from build123d import *

# Parameters (mm, degrees)
BOSS_EXTRUDE1_DEPTH            = 40.64
F_31_0_12_DIAMETER_HOLE2_D     = 3.048
F_31_0_12_DIAMETER_HOLE2_DEPTH = 12.7
F_31_0_12_DIAMETER_HOLE2_TIP   = 0.915711583
F_31_0_12_DIAMETER_HOLE1_D     = 3.048
F_31_0_12_DIAMETER_HOLE1_DEPTH = 12.7
F_31_0_12_DIAMETER_HOLE1_TIP   = 0.915711583
CHAMFER1_SIZE                  = 31.75


with BuildPart() as part:
    # Sketch1 → Boss-Extrude1 (new, symmetric)
    with BuildSketch(Plane.XY):
        Polygon((48.0568, 17.74825), (-48.0568, 17.74825), (-48.0568, -17.74825), (-40.132, -17.74825), (-40.132, 12.98575), (40.132, 12.98575), (40.132, -17.74825), (48.0568, -17.74825), align=None)
    extrude(amount=BOSS_EXTRUDE1_DEPTH, both=True)

    # #31 (0.12) Diameter Hole2
    with Locations(Plane(origin=(0, -17.74825, 0), x_dir=(-1, 0, 0), z_dir=(0, -1, 0))):
        with Locations((-44.0944, 0), (44.0944, 0)):
            Hole(F_31_0_12_DIAMETER_HOLE2_D / 2, depth=F_31_0_12_DIAMETER_HOLE2_DEPTH)
            with Locations((0, 0, -(F_31_0_12_DIAMETER_HOLE2_DEPTH + F_31_0_12_DIAMETER_HOLE2_TIP / 2))):  # 118° drill point
                Cone(0, F_31_0_12_DIAMETER_HOLE2_D / 2, F_31_0_12_DIAMETER_HOLE2_TIP, mode=Mode.SUBTRACT)

    # #31 (0.12) Diameter Hole1
    with Locations(Plane(origin=(0, 17.74825, 0), x_dir=(1, 0, 0), z_dir=(0, 1, 0))):
        with Locations((0, -36.83), (0, 36.83)):
            Hole(F_31_0_12_DIAMETER_HOLE1_D / 2, depth=F_31_0_12_DIAMETER_HOLE1_DEPTH)
            with Locations((0, 0, -(F_31_0_12_DIAMETER_HOLE1_DEPTH + F_31_0_12_DIAMETER_HOLE1_TIP / 2))):  # 118° drill point
                Cone(0, F_31_0_12_DIAMETER_HOLE1_D / 2, F_31_0_12_DIAMETER_HOLE1_TIP, mode=Mode.SUBTRACT)

    # Chamfer1
    chamfer1_edges = [part.edges().sort_by_distance(p)[0] for p in [
        (-48.0568, 0, 40.64),
        (-48.0568, 0, -40.64),
        (48.0568, 0, -40.64),
        (48.0568, 0, 40.64),
    ]]
    chamfer(chamfer1_edges, length=CHAMFER1_SIZE)


solid = part.part
Work out the finished part from the listing and answer in its coordinate system (mm). A direction names the side the tool comes from. Coordinates: 2 decimals unless noted, no trailing zeros. Write each loop counter-clockwise with the first axis right and the second up, starting at its lowest first coordinate (ties: lowest second). Pieces come first, ordered by that corner, then holes. Notation, with made-up numbers: M 19,-24.5 L 43,-24.5 A24 ccw 43,-10.5 Z; hole C 59,63.5 d7. An arc over 180 degrees is marked long. Use one line per item in the form item = value. Start each with the question number.
1. A tool of negligible diameter and unlimited length cuts with its end or side. For faces 1 (the face through (-40.132, -3, 0)), 2 (the face through (40.339, 2.547, 16.608)), 3 (the face through (-45.617, -11.309, -0.067)), from which of +Z, -Z, +X, -X, +Y, -Y can it reach the whole face along a straight path? Write none if from no direction.
2. Each of these flat-tipped pins is pushed along its axis until it touches: P1, Ø3, axis at x = 37.5, y = 13.5, coming from the -Z side; P2, Ø10, axis at x = -17, z = 7.5, coming from the -Y side; P3, Ø6, axis at y = -1.5, z = -17, coming from the -X side; P4, Ø2.5, axis at x = 0, z = 36.83, coming from the +Y side. Where does it stop, or does it pass through?
3. The part is cut by section C-C (z = 36.83). Give the vertices of the cut face in (x, y).
4. The part is cut by section D-D (z = 15). Give the vertices of the cut face in (x, y), plus the area to 3 significant figures.
5. The part is cut by section A-A (x = 0). Give the vertices of the cut face in (y, z).
6. The mould has two halves that part along Z. Classify faces 4 (the face through (0.2, 15.33, -38.34)), 5 (the face through (1, 17.748, 1)), 6 (the face through (-40.487, 4.027, -16.459)): released by +Z, released by -Z, zero draft, split by the parting line, or undercut.
7. Straight lines are drawn through the part: probe 1 along Z at (x, y) = (0, 16.4); probe 2 along X at (y, z) = (-11, 2); probe 3 along Y at (x, z) = (-32, 12.5). For each, find the intervals that lie inside material, in ascending order. Write a range as from..to.
8. The part is cut by section B-B (y = 1). Give the vertices of the cut face in (x, z), plus the area to 3 significant figures.
Evaluation:
q1.face_1 = +Z, -Z, -Y
q1.face_2 = +Z, +X, +Y, -Y
q1.face_3 = -Y
q2.P1 = -20.95
q2.P2 = 12.99
q2.P3 = -42.95
q2.P4 = through
q3.outline = M -20.12,12.99 L -1.52,12.99 L -1.52,17.75 L -20.12,17.75 Z; M 1.52,12.99 L 20.12,12.99 L 20.12,17.75 L 1.52,17.75 Z
q4.outline = M -41.95,-17.75 L -40.13,-17.75 L -40.13,12.99 L 40.13,12.99 L 40.13,-17.75 L 41.95,-17.75 L 41.95,17.75 L -41.95,17.75 Z
q4.area = 511 mm^2
q5.outline = M 12.99,-40.64 L 17.75,-40.64 L 17.75,-38.35 L 12.99,-38.35 Z; M 12.99,-35.31 L 17.75,-35.31 L 17.75,35.31 L 12.99,35.31 Z; M 12.99,38.35 L 17.75,38.35 L 17.75,40.64 L 12.99,40.64 Z
q6.face_4 = undercut
q6.face_5 = zero draft
q6.face_6 = released by -Z
q7.probe_1 = -40.64..-38.35, -35.31..35.31, 38.35..40.64
q7.probe_2 = -48.06..-40.13, 40.13..48.06
q7.probe_3 = 12.99..17.75
q8.outline = M -48.06,-8.89 L -40.13,-16.81 L -40.13,16.81 L -48.06,8.89 Z; M 40.13,-16.81 L 48.06,-8.89 L 48.06,8.89 L 40.13,16.81 Z
q8.area = 407 mm^2
